Model file for the job. Use its own axes, mm. A direction names the side the tool comes from. Give positions to 0.01 mm unless a question says otherwise; leave off trailing zeros. Order: outer loops, then holes, each group sorted by start corner. A loop starts at its lowest first (then second) coordinate and runs counter-clockwise, first axis right, second up. Notation, with made-up numbers: (47, 76) -> (55, 76) arc R24 cw to (55, 105) -> close; hole circle Ø7 at (23, 40). An arc over 180 degrees is marked (long way). Answer in a Markdown table with one row per item. Add a question column.
from build123d import *

# Parameters (mm, degrees)
SKETCH_R      = 16
SKETCH_R_2    = 2.8
SKETCH_R_3    = 3.5
PAD_DEPTH     = 3
SKETCH001_R   = 16
SKETCH001_R_2 = 5.2
SKETCH001_R_3 = 1.8
PAD001_DEPTH  = 3


with BuildPart() as pad:
    # Sketch → Pad (new body)
    with BuildSketch(Plane.XY):
        Circle(SKETCH_R)
        with Locations((-6, 0)):
            Circle(SKETCH_R_2, mode=Mode.SUBTRACT)
        with Locations((6, 0)):
            Circle(SKETCH_R_2, mode=Mode.SUBTRACT)
        with Locations((0, 10)):
            Circle(SKETCH_R_3, mode=Mode.SUBTRACT)
        with Locations((0, -10)):
            Circle(SKETCH_R_3, mode=Mode.SUBTRACT)
    extrude(amount=PAD_DEPTH)


with BuildPart() as fusion:
    # Sketch001 → Pad001 (new body)
    with BuildSketch(Plane.XY.offset(3)):
        Circle(SKETCH001_R)
        with Locations((-6, 0)):
            Circle(SKETCH001_R_2, mode=Mode.SUBTRACT)
        with Locations((6, 0)):
            Circle(SKETCH001_R_2, mode=Mode.SUBTRACT)
        with Locations((0, 10)):
            Circle(SKETCH001_R_3, mode=Mode.SUBTRACT)
        with Locations((0, -10)):
            Circle(SKETCH001_R_3, mode=Mode.SUBTRACT)
    extrude(amount=PAD001_DEPTH)

    # Fusion: union Pad
    add(pad.part)


solid = fusion.part
Item 1: Saw through at A-A on y = 0. List the corners of the cut face in (x, z).
Item 2: Which spindle directions (+Z, -Z, +X, -X, +Y, -Y) get a long thin tool onto all of the face, cutting with end or side? Do faces 4 (the cylindrical face through (-0.759, 6.583, 1.479)), 5 (the cylindrical face through (0.805, 0.229, 4.479)), 6 (the cylindrical face through (3.2, 0.1, 1.5)). Say none if no direction does.
Item 3: Saw through at C-C on y = 10. List the corners of the cut face in (x, z), plus the area to 3 significant figures.
Item 4: Wall check: line 1 (Y direction, x = 0, z = 4.15); line 2 (X direction, y = -4, z = 4.3); line 3 (Y direction, x = -2, z = 0.5). Give the ranges that are in metal, low to high.
Item 5: Pin check, flat tips, straight feed: pin 1 Ø1.5 at (x, z) = (-5.5, 5) entering from +Y; pin 2 Ø4 at (x, y) = (0, 10) entering from -Z; pin 3 Ø9.5 at (x, y) = (6, 0) entering from +Z. Stop position of each tip, or through.
Item 6: Saw through at B-B on x = 0. List the corners of the cut face in (y, z).
Item 7: Two-plate mould, pull along Y, no slides. Class faces 1 (the flat face through (0, 0, 6)), 2 (the cylindrical face through (-3.33, 0.84, 1.48)), 3 (the cylindrical face through (-3.47, -15.62, 2.96)): pulls with the +Y half, pulls with the -Y half, needs draft (parallel to the pull), parting line crosses it, or undercut.
Item 8: Saw through at D-D on x = 5.5. List the corners of the cut face in (y, z) (3 decimals).
Evaluation:
| question | item | result |
|---|---|---|
| 1 | outline | (-16, 0) -> (-8.8, 0) -> (-8.8, 3) -> (-11.2, 3) -> (-11.2, 6) -> (-16, 6) -> close; (-3.2, 0) -> (3.2, 0) -> (3.2, 3) -> (0.8, 3) -> (0.8, 6) -> (-0.8, 6) -> (-0.8, 3) -> (-3.2, 3) -> close; (8.8, 0) -> (16, 0) -> (16, 6) -> (11.2, 6) -> (11.2, 3) -> (8.8, 3) -> close |
| 2 | face 4 | -Z |
| 2 | face 5 | +Z |
| 2 | face 6 | +Z, -Z |
| 3 | outline | (-12.49, 0) -> (-3.5, 0) -> (-3.5, 3) -> (-1.8, 3) -> (-1.8, 6) -> (-12.49, 6) -> close; (1.8, 3) -> (3.5, 3) -> (3.5, 0) -> (12.49, 0) -> (12.49, 6) -> (1.8, 6) -> close |
| 3 | area | 118 mm2 |
| 4 | line 1 | y = -16 to -11.8, -8.2 to 8.2, 11.8 to 16 |
| 4 | line 2 | x = -15.49 to -9.32, -2.68 to 2.68, 9.32 to 15.49 |
| 4 | line 3 | y = -15.87 to -12.87, -7.13 to 7.13, 12.87 to 15.87 |
| 5 | pin 1 | stops at y = 15.28 |
| 5 | pin 2 | stops at z = 3 |
| 5 | pin 3 | stops at z = 3 |
| 6 | outline | (-16, 0) -> (-13.5, 0) -> (-13.5, 3) -> (-11.8, 3) -> (-11.8, 6) -> (-16, 6) -> close; (-8.2, 3) -> (-6.5, 3) -> (-6.5, 0) -> (6.5, 0) -> (6.5, 3) -> (8.2, 3) -> (8.2, 6) -> (-8.2, 6) -> close; (11.8, 3) -> (13.5, 3) -> (13.5, 0) -> (16, 0) -> (16, 6) -> (11.8, 6) -> close |
| 7 | face 1 | needs draft |
| 7 | face 2 | undercut |
| 7 | face 3 | parting line crosses it |
| 8 | outline | (-15.025, 0) -> (-2.755, 0) -> (-2.755, 3) -> (-5.176, 3) -> (-5.176, 6) -> (-15.025, 6) -> close; (2.755, 0) -> (15.025, 0) -> (15.025, 6) -> (5.176, 6) -> (5.176, 3) -> (2.755, 3) -> close |
